```python
from build123d import *

# Parameters (mm, degrees)
F1_DEPTH = 125
F2_R     = 50
F3_R     = 10
F4_T     = -2.5


with BuildPart() as f1:
    # F0 (on Front) → F1 (new body, symmetric)
    with BuildSketch(Plane.XZ):
        with BuildLine():
            Line((98.826939, 35.839786), (18.805769, 60.651406))
            ThreePointArc((18.805769, 60.651406), (-63.5, 0), (18.805769, -60.651406))
            Line((18.805769, -60.651406), (98.826939, -35.839786))
            ThreePointArc((98.826939, -35.839786), (177.5, 0), (98.826939, 35.839786))
        make_face()
    extrude(amount=F1_DEPTH, both=True)

    # F2
    f2_edges = [f1.edges().sort_by_distance(p)[0] for p in [
        (98.826939, 0, 35.839786),
        (98.826939, 0, -35.839786),
    ]]
    fillet(f2_edges, radius=F2_R)

    # F3
    f3_edges = [f1.edges().sort_by_distance(p)[0] for p in [
        (48.352342, 125, -51.490101),
    ]]
    fillet(f3_edges, radius=F3_R)

    # F4
    f4_openings = [f1.faces().sort_by_distance(p)[0] for p in [
        (49.834111, -125, 0),
    ]]
    offset(amount=F4_T, openings=f4_openings)


solid = f1.part
```
Here's how the part is built. I have some questions about the finished solid (model axes, mm). A direction names the side the tool comes from. Round coordinates to 2 decimals unless told otherwise and drop trailing zeros. Order: outer loops, then holes, each group sorted by start corner. A loop starts at its lowest first (then second) coordinate and runs counter-clockwise, first axis right, second up. Notation, with made-up numbers: M 57,31.5 L 101,31.5 A21 ccw 101,53.5 Z; hole C 2,-39.75 d3. An arc over 180 degrees is marked long. Answer in a Markdown table with one row per item.
Item 1: I'm going to push flat-ended pins straight in: pin 1 (6 mm diameter, centred on x = 119.5, y = -38.5, fed in from +Z); pin 2 (6 mm diameter, centred on x = 20.5, y = -48.5, fed in from +Z); pin 3 (5 mm diameter, centred on x = 49.5, y = -72.5, fed in from -Z). Where does each tip first touch, or does it pass through?
A:
| item | result |
|---|---|
| pin 1 | stops at z = 46.9 |
| pin 2 | stops at z = 61.04 |
| pin 3 | stops at z = -51.91 |
Item 2: If I drill on L1, parallel to Z at x = 130, y = -43; L2, parallel to Z at x = 0, y = -33; L3, parallel to X at y = -60.5, z = 23.5, over which ranges is the centre line in solid material (lowest first)? Write a range as from..to.
A:
| item | result |
|---|---|
| L1 | z = -47.5..-45, 45..47.5 |
| L2 | z = -63.5..-61, 61..63.5 |
| L3 | x = -58.99..-56.29, 168.38..171.28 |
Item 3: For faces 1 (the face through (47.875, 122.148, -48.49)), 2 (the face through (47.048, 122.148, 48.746)), 3 (the face through (47.94, -6.68, -51.62)), 4 (the face through (95.371, -3.32, -37.653)), 5 (the face through (48.77, -6.68, 51.36)), which set-ups out of +Z, -Z, +X, -X, +Y, -Y let a thin tool reach every point of the face, with its end or its side?
A:
| item | result |
|---|---|
| face 1 | -Z, +Y |
| face 2 | +Z, +Y |
| face 3 | -Z, +Y, -Y |
| face 4 | -Y |
| face 5 | +Z, +Y, -Y |
Item 4: Imagine slicing it at A-A, the plane y = -105. Write out the boundary of the cut face in (x, z), and give its area (3 significant figures).
A:
| item | result |
|---|---|
| outline | M 18.81,-60.65 L 77.9,-42.33 A50 cw 111.83,-43.89 A47.5 ccw long 111.83,43.89 A50 cw 77.9,42.33 L 18.81,60.65 A63.5 ccw long Z; hole M 18.07,-58.26 L 77.16,-39.94 A52.5 cw 112.79,-41.58 A45 ccw long 112.79,41.58 A52.5 cw 77.16,39.94 L 18.07,58.26 A61 ccw long Z |
| area | 1,520 mm2 |
Item 5: Thinking about a two-plate mould opening in X: for faces 6 (the face through (55, 122.5, 1)), 7 (the face through (56, -125, 47)), 8 (the face through (-63.48, -6.68, 1.66)), which applies, +X half, -X half, draft (parallel to the pull), parting line (faces both ways), or undercut?
A:
| item | result |
|---|---|
| face 6 | undercut |
| face 7 | draft |
| face 8 | parting line |
Item 6: Imagine slicing it at B-B, the plane z = 0. Write out the boundary of the cut face in (x, y).
A:
| item | result |
|---|---|
| outline | M -63.5,-125 L -61,-125 L -61,115 A7.5 cw -53.5,122.5 L 167.5,122.5 A7.5 cw 175,115 L 175,-125 L 177.5,-125 L 177.5,115 A10 ccw 167.5,125 L -53.5,125 A10 ccw -63.5,115 Z |
